```python
from build123d import *

# Parameters (mm, degrees)
SKETCH1_W            = 101.6
SKETCH1_H            = 50.8
BOSS_EXTRUDE1_DEPTH  = 228.6
SKETCH2_W            = 96.52
SKETCH2_H            = 172.72
CUT_EXTRUDE1_DEPTH   = 50.8
BOSS_EXTRUDE2_DEPTH  = 50.8
BOSS_EXTRUDE3_DEPTH  = 101.6
SKETCH13_W           = 96.52
SKETCH13_H           = 25.4
CUT_EXTRUDE2_DEPTH   = 50.8
SKETCH14_W           = 96.52
SKETCH14_H           = 25.4
CUT_EXTRUDE3_DEPTH   = 50.8
SKETCH15_W           = 96.52
SKETCH15_H           = 50.8
CUT_EXTRUDE6_DEPTH   = 6.35
SKETCH16_W           = 96.52
SKETCH16_H           = 45.72
CUT_EXTRUDE7_DEPTH   = 3.175
SKETCH17_W           = 101.6
SKETCH17_H           = 25.4
CUT_EXTRUDE8_DEPTH   = 228.6
SKETCH20_W           = 6.35
SKETCH20_H           = 12.7
BOSS_EXTRUDE5_DEPTH  = 101.6
SKETCH24_W           = 12.7
SKETCH24_H           = 6.35
BOSS_EXTRUDE8_DEPTH  = 19.05
SKETCH26_W           = 12.7
SKETCH26_H           = 6.35
BOSS_EXTRUDE10_DEPTH = 19.05
SKETCH27_W           = 12.7
SKETCH27_H           = 6.35
BOSS_EXTRUDE11_DEPTH = 19.05
SKETCH33_W           = 96.52
SKETCH33_H           = 2.54
BOSS_EXTRUDE13_DEPTH = 2.54
SKETCH34_W           = 96.52
SKETCH34_H           = 2.54
BOSS_EXTRUDE17_DEPTH = 2.54
SKETCH36_W           = 218.44
SKETCH36_H           = 2.54
BOSS_EXTRUDE18_DEPTH = 2.54
SKETCH37_W           = 218.44
SKETCH37_H           = 2.54
BOSS_EXTRUDE19_DEPTH = 2.54
SKETCH45_W           = 13.208
SKETCH45_H           = 10.16
CUT_EXTRUDE19_DEPTH  = 6.35
CUT_EXTRUDE22_START  = -101.6
CUT_EXTRUDE22_DEPTH  = 101.6
SKETCH60_R           = 4.445
CUT_EXTRUDE23_DEPTH  = 2.54
SKETCH61_R           = 4.445
CUT_EXTRUDE24_DEPTH  = 2.54
SKETCH64_W           = 95.25
SKETCH64_H           = 6.35
BOSS_EXTRUDE33_DEPTH = 6.35


# Read off the part's stored shape, not the designer's step: Cut-Extrude22
with BuildPart() as part:
    # Sketch1 → Boss-Extrude1 (new body)
    with BuildSketch(Plane.XY):
        Rectangle(SKETCH1_W, SKETCH1_H)
    extrude(amount=-BOSS_EXTRUDE1_DEPTH)

    # Sketch2 → Cut-Extrude1 (cut)
    with BuildSketch(Plane(origin=(0, 25.4, 0), x_dir=(1, 0, 0), z_dir=(0, 1, 0))):
        with Locations((0, 114.3)):
            Rectangle(SKETCH2_W, SKETCH2_H)
    extrude(amount=-CUT_EXTRUDE1_DEPTH, mode=Mode.SUBTRACT)

    # Sketch3 → Boss-Extrude2 (add)
    with BuildSketch(Plane(origin=(0, 25.4, 0), x_dir=(1, 0, 0), z_dir=(0, 1, 0))):
        Polygon((48.26, 73.001295984), (48.26, 79.351295984), (-48.26, 79.351295984), (-48.26, 73.001295984), (0, 73.001295984), align=None)
    extrude(amount=-BOSS_EXTRUDE2_DEPTH)

    # Sketch11 → Boss-Extrude3 (add)
    with BuildSketch(Plane.ZY.offset(50.8)):
        Polygon((-79.351295984, 25.4), (-113.622558301, 63.5), (-106.756614843, 63.363382999), (-73.001295984, 25.4), align=None)
    extrude(amount=-BOSS_EXTRUDE3_DEPTH)

    # Sketch13 → Cut-Extrude2 (cut)
    with BuildSketch(Plane(origin=(0, 25.4, 0), x_dir=(1, 0, 0), z_dir=(0, 1, 0))):
        with Locations((0, 213.36)):
            Rectangle(SKETCH13_W, SKETCH13_H)
    extrude(amount=-CUT_EXTRUDE2_DEPTH, mode=Mode.SUBTRACT)

    # Sketch14 → Cut-Extrude3 (cut)
    with BuildSketch(Plane(origin=(0, 25.4, 0), x_dir=(1, 0, 0), z_dir=(0, 1, 0))):
        with Locations((0, 15.24)):
            Rectangle(SKETCH14_W, SKETCH14_H)
    extrude(amount=-CUT_EXTRUDE3_DEPTH, mode=Mode.SUBTRACT)

    # Sketch15 → Cut-Extrude6 (cut)
    with BuildSketch(Plane.XY.offset(-73.001295984)):
        Rectangle(SKETCH15_W, SKETCH15_H)
    extrude(amount=-CUT_EXTRUDE6_DEPTH, mode=Mode.SUBTRACT)

    # Sketch16 → Cut-Extrude7 (cut)
    with BuildSketch(Plane(origin=(0, -25.035409247, -28.156416881), x_dir=(1, 0, 0), z_dir=(0, 0.6644747806949454, 0.7473106889509907))):
        with Locations((0, 92.889211639)):
            Rectangle(SKETCH16_W, SKETCH16_H)
    extrude(amount=-CUT_EXTRUDE7_DEPTH, mode=Mode.SUBTRACT)

    # Sketch17 → Cut-Extrude8 (cut)
    with BuildSketch(Plane.XY):
        with Locations((0, -12.7)):
            Rectangle(SKETCH17_W, SKETCH17_H)
    extrude(amount=-CUT_EXTRUDE8_DEPTH, mode=Mode.SUBTRACT)

    # Sketch20 → Boss-Extrude5 (add)
    with BuildSketch(Plane.ZY.offset(50.8)):
        with Locations((-174.625, 6.35)):
            Rectangle(SKETCH20_W, SKETCH20_H)
    extrude(amount=-BOSS_EXTRUDE5_DEPTH)

    # Sketch24 → Boss-Extrude8 (add)
    with BuildSketch(Plane.XZ):
        with Locations((44.45, -76.176295984)):
            Rectangle(SKETCH24_W, SKETCH24_H)
    extrude(amount=BOSS_EXTRUDE8_DEPTH)

    # Sketch26 → Boss-Extrude10 (add)
    with BuildSketch(Plane.XZ):
        with Locations((-44.45, -174.625)):
            Rectangle(SKETCH26_W, SKETCH26_H)
    extrude(amount=BOSS_EXTRUDE10_DEPTH)

    # Sketch27 → Boss-Extrude11 (add)
    with BuildSketch(Plane.XZ):
        with Locations((44.45, -174.625)):
            Rectangle(SKETCH27_W, SKETCH27_H)
    extrude(amount=BOSS_EXTRUDE11_DEPTH)

    # Sketch33 → Boss-Extrude13 (add)
    with BuildSketch(Plane(origin=(0, 0, -2.54), x_dir=(-1, 0, 0), z_dir=(0, 0, -1))):
        with Locations((0, 12.7)):
            Rectangle(SKETCH33_W, SKETCH33_H)
    extrude(amount=BOSS_EXTRUDE13_DEPTH)

    # Sketch34 → Boss-Extrude17 (add)
    with BuildSketch(Plane.XY.offset(-226.06)):
        with Locations((0, 12.7)):
            Rectangle(SKETCH34_W, SKETCH34_H)
    extrude(amount=BOSS_EXTRUDE17_DEPTH)

    # Sketch36 → Boss-Extrude18 (add)
    with BuildSketch(Plane(origin=(-48.26, 0, 0), x_dir=(0, 0, -1), z_dir=(1, 0, 0))):
        with Locations((114.3, 12.7)):
            Rectangle(SKETCH36_W, SKETCH36_H)
    extrude(amount=BOSS_EXTRUDE18_DEPTH)

    # Sketch37 → Boss-Extrude19 (add)
    with BuildSketch(Plane.ZY.offset(-48.26)):
        with Locations((-114.3, 12.7)):
            Rectangle(SKETCH37_W, SKETCH37_H)
    extrude(amount=BOSS_EXTRUDE19_DEPTH)

    # Sketch45 → Cut-Extrude19 (cut)
    with BuildSketch(Plane.XY):
        with Locations((37.933039121, 12.7)):
            Rectangle(SKETCH45_W, SKETCH45_H)
        with Locations((-37.933039121, 12.7)):
            Rectangle(SKETCH45_W, SKETCH45_H)
    extrude(amount=-CUT_EXTRUDE19_DEPTH, mode=Mode.SUBTRACT)

    # Cut-Extrude22 outline → Cut-Extrude22 (cut)
    with BuildSketch(Plane.ZY.offset(50.8).offset(CUT_EXTRUDE22_START)):
        Polygon((-73.001295984, 0), (0, 0), (0, 25.4), (-228.6, 25.4), (-228.6, 0), (-177.8, 0), (-177.8, -19.05), (-171.45, -19.05), (-171.45, 0), (-79.351295984, 0), (-79.351295984, -19.05), (-73.001295984, -19.05), align=None)
    extrude(amount=CUT_EXTRUDE22_DEPTH, mode=Mode.SUBTRACT)

    # Sketch60 → Cut-Extrude23 (cut)
    with BuildSketch(Plane(origin=(0, -27.145116675, -30.529128319), x_dir=(1, 0, 0), z_dir=(0, 0.6644747806949455, 0.7473106889509905))):
        with Locations(Location((38.1, 77.014211639, 0), (0, 0, 270))):
            Circle(SKETCH60_R)
    extrude(amount=-CUT_EXTRUDE23_DEPTH, mode=Mode.SUBTRACT)

    # Sketch61 → Cut-Extrude24 (cut)
    with BuildSketch(Plane(origin=(0, -27.145116675, -30.529128319), x_dir=(1, 0, 0), z_dir=(0, 0.6644747806949455, 0.7473106889509905))):
        with Locations(Location((-2.54, 77.014211639, 0), (0, 0, 270))):
            Circle(SKETCH61_R)
    extrude(amount=-CUT_EXTRUDE24_DEPTH, mode=Mode.SUBTRACT)

    # Sketch64 → Boss-Extrude33 (add)
    with BuildSketch(Plane(origin=(0, 25.4, 0), x_dir=(-1, 0, 0), z_dir=(0, -1, 0))):
        with Locations((0, 76.176295984)):
            Rectangle(SKETCH64_W, SKETCH64_H)
    extrude(amount=BOSS_EXTRUDE33_DEPTH)


solid = part.part
```
For this review, take the finished solid that the model builds, in its own axes (mm). A direction names the side the tool comes from. Coordinates: 2 decimals unless noted, no trailing zeros. Loops run counter-clockwise (first coordinate to the right, second up) from the corner with the lowest first, then second, coordinate; pieces in that order, holes last.
1. Mouldability with a two-part tool opening along Y and no side actions: class faces 1 (the flat face through (-47.625, 22, -76)), 2 (the flat face through (-0.676, 60.425, -106.239)), 3 (the flat face through (49, 25.4, -76)) as +Y half, -Y half, draft (parallel to the pull), parting line (faces both ways), or undercut.
2. For line 1 (X direction, y = 57.5, z = -104); line 2 (Y direction, x = 1, z = -77); line 3 (X direction, y = 24, z = -76) (3 decimals), list the stretches that pass through material, from the lowest coordinate up.
3. For faces 4 (the flat face through (47.625, 22, -76)), 5 (the flat face through (1, 22, -79.351)), 6 (the flat face through (-0.7, 26.4, -75.7)), list the 3-axis set-ups (+Z, -Z, +X, -X, +Y, -Y) from which the entire face can be reached by the end or side of a thin tool; tool diameter is ignored.
4. Add section A-A, the plane x = -0.5. Give the boundary of the cut face in (y, z).
5. Add section C-C, the plane y = 48.5. Give the boundary of the cut face in (x, z).
6. Add section D-D, the plane z = -81.5. Count the separate pieces of the cut face and the enclosed holes in it, then the cut area to 3 significant figures.
7. Insertion check: P1, Ø1.5, axis at x = 34, y = 46.5, coming from the +Z side; P2, Ø3, axis at y = 21, z = -76, coming from the -X side (3 decimals); P3, Ø1.6, axis at x = -50, z = -75, coming from the -Y side. Each pin has a flat end and moves straight along its axis. Give the tip position at first contact, or say it passes through.
8. Add section B-B, the plane z = -101. Give the boundary of the cut face in (x, y).
Result:
1. face 1: draft
1. face 2: undercut
1. face 3: -Y half
2. line 1: x = -50.8 to -48.26, 48.26 to 50.8
2. line 2: y = 19.05 to 25.4
2. line 3: x = -47.625 to 47.625
3. face 4: +Z, -Z, +X, -Y
3. face 5: -Z, +X, -X, -Y
3. face 6: +Y
4. outline: (19.05, -79.35) - (25.4, -79.35) - (26.41, -80.26) - (27.46, -79.08) - (25.4, -77.25) - (25.4, -76.82) - (27.3, -74.69) - (25.4, -73) - (19.05, -73) - close; (32.28, -85.54) - (63.5, -113.62) - (63.36, -106.76) - (61.47, -105.07) - (59.36, -107.44) - (33.36, -84.33) - close
5. outline: (-50.8, -100.13) - (50.8, -100.13) - (50.8, -93.54) - (48.26, -93.54) - (48.26, -97.79) - (-48.26, -97.79) - (-48.26, -93.54) - (-50.8, -93.54) - close
6. separate pieces: 3
6. enclosed holes: 0
6. area: 227 mm2
7. P1: stops at z = -95.34
7. P2: stops at x = -47.625
7. P3: stops at y = 25.4
8. outline: (-50.8, 49.47) - (50.8, 49.47) - (50.8, 56.89) - (48.26, 56.89) - (48.26, 52.11) - (-48.26, 52.11) - (-48.26, 56.89) - (-50.8, 56.89) - close
